Part model, mm, in its own coordinate system. Give positions to 0.01 mm unless a question says otherwise; leave off trailing zeros. Loops run counter-clockwise (first coordinate to the right, second up) from the corner with the lowest first, then second, coordinate; pieces in that order, holes last. Notation, with made-up numbers: (-17.5, 83) -> (7.5, 83) arc R19 ccw to (7.5, 112) -> close; hole circle Ø3 at (59, 41.5). An arc over 180 degrees is marked (long way). Write item = value, one per line.
from build123d import *

# Parameters (mm, degrees)
SKETCH1_W           = 76.2
SKETCH1_H           = 76.2
BOSS_EXTRUDE1_DEPTH = 6.35
SKETCH3_R           = 0.396875
CUT_EXTRUDE2_DEPTH  = 7.35
SKETCH4_R           = 1.5875
CUT_EXTRUDE3_DEPTH  = 7.35


with BuildPart() as part:
    # Sketch1 → Boss-Extrude1 (new body)
    with BuildSketch(Plane.XY):
        with Locations((38.1, 38.1)):
            Rectangle(SKETCH1_W, SKETCH1_H)
    extrude(amount=BOSS_EXTRUDE1_DEPTH)

    # Sketch3 → Cut-Extrude2 (cut, through all)
    with BuildSketch(Plane.XY.offset(6.35)):
        with Locations((49.403, 49.403)):
            Circle(SKETCH3_R)
        with Locations((26.797, 49.403)):
            Circle(SKETCH3_R)
        with Locations((26.797, 26.797)):
            Circle(SKETCH3_R)
        with Locations((49.403, 26.797)):
            Circle(SKETCH3_R)
    extrude(amount=-CUT_EXTRUDE2_DEPTH, mode=Mode.SUBTRACT)

    # Sketch4 → Cut-Extrude3 (cut, through all)
    with BuildSketch(Plane(origin=(0, 0, 0), x_dir=(-1, 0, 0), z_dir=(0, 0, -1))):
        with Locations((-6.35, 69.85)):
            Circle(SKETCH4_R)
        with Locations((-6.35, 6.35)):
            Circle(SKETCH4_R)
        with Locations((-69.85, 69.85)):
            Circle(SKETCH4_R)
        with Locations((-69.85, 6.35)):
            Circle(SKETCH4_R)
    extrude(amount=-CUT_EXTRUDE3_DEPTH, mode=Mode.SUBTRACT)


solid = part.part
1) Drop a flat-ended pin along its axis: P1, Ø12, axis at x = 55, y = 50.5, coming from the -Z side. Give the stop position or say it passes through.
Resolved:
P1 = 0
2) Slice it at A-A, the plane x = 69.85. List the corners of the cut face in (y, z), and give its area (3 significant figures).
Resolved:
outline = (0, 0) -> (4.76, 0) -> (4.76, 6.35) -> (0, 6.35) -> close; (7.94, 0) -> (68.26, 0) -> (68.26, 6.35) -> (7.94, 6.35) -> close; (71.44, 0) -> (76.2, 0) -> (76.2, 6.35) -> (71.44, 6.35) -> close
area = 444 mm²
3) Drill centre lines: line 1 along Y through (x, z) = (6.35, 2.5); line 2 along Y through (x, z) = (7, 1.75). Where is each one in solid material? Low to high. Write a range as [from, to].
Resolved:
line_1 = [0, 4.76], [7.94, 68.26], [71.44, 76.2]
line_2 = [0, 4.9], [7.8, 68.4], [71.3, 76.2]
